Source: CAD feature listing. Evaluate the final solid. Frame: model axes, mm. A direction names the side the tool comes from. Coordinates: 2 decimals unless noted, no trailing zeros. Write each loop counter-clockwise with the first axis right and the second up, starting at its lowest first coordinate (ties: lowest second). Pieces come first, ordered by that corner, then holes. Notation, with made-up numbers: (-24.75, 11) -> (-20.75, 11) arc R17 cw to (-20.75, 40) -> close; hole circle Ø4 at (80.25, 82.5). An arc over 180 degrees is marked (long way). One line per item, written item: value. Start each with the question number.
1. Access query for faces 4 (the flat face through (25, 21, 0)), 5 (the flat face through (43, 31, 2)), 6 (the flat face through (46, 30, 35)). Directions: +Z, -Z, +X, -X, +Y, -Y. A direction counts if a zero-diameter tool reaches every point of the face in a straight line with its end or side. Return the directions, or none.
2. Section query C-C, the plane z = 10.65. Output: boundary loops of the cut face in (x, y) (3 decimals), and give its area (3 significant figures).
3. Section query D-D, the plane z = 3. Output: boundary loops of the cut face in (x, y).
4. Section query A-A, the plane y = 5.65. Output: boundary loops of the cut face in (x, z) (3 decimals).
5. Line query: line 1 (Z direction, x = 48.6, y = 5.65) (3 decimals); line 2 (Y direction, x = 48, z = 26); line 3 (Z direction, x = 7.5, y = 32). Output: solid intervals per line, ascending.
6. First-contact query: P1, Ø8, axis at y = 4.5, z = 40.5, coming from the -X side; P2, Ø12.5, axis at x = 18.5, y = 13.5, coming from the +Z side; P3, Ø3, axis at x = 42, y = 32.65, coming from the -Z side; P4, Ø1.7, axis at x = 4.5, y = 11, coming from the +Z side. Flat tips, straight axial feed; report the tip coordinate or a pass-through.
7. Mould query, pull axis Y, two halves, no side actions, for faces 1 (the cylindrical face through (47.97, 35.9, 40.21)), 2 (the cylindrical face through (48.03, 40.8, 45.87)), 3 (the flat face through (0, 21, 2)). Classes: released by +Y, released by -Y, zero draft, split by the parting line, or undercut.
8. Section query B-B, the plane x = 42. Output: boundary loops of the cut face in (y, z) (3 decimals), and give its area (4 significant figures).
from build123d import *

# Parameters (mm, degrees)
F0_W     = 50
F0_H     = 42.3
F0_R     = 2.8
F0_R_2   = 1.625
F1_DEPTH = 4
F2_R     = 2.8
F2_R_2   = 1.625
F3_DEPTH = 2
F4_W     = 4
F4_H     = 42.3
F5_DEPTH = 43.3
F6_R     = 12
F6_R_2   = 1.625
F7_DEPTH = 25
F8_R     = 5


with BuildPart() as f1:
    # F0 (on Top) → F1 (new body)
    with BuildSketch(Plane.XY):
        with Locations((25, 21.15)):
            Rectangle(F0_W, F0_H)
        with Locations((4, 9.65)):
            Circle(F0_R, mode=Mode.SUBTRACT)
        with Locations((42, 32.65)):
            Circle(F0_R, mode=Mode.SUBTRACT)
        with Locations((42, 32.65)):
            Circle(F0_R)
        with Locations((42, 32.65)):
            Circle(F0_R_2, mode=Mode.SUBTRACT)
        with Locations((4, 9.65)):
            Circle(F0_R)
        with Locations((4, 9.65)):
            Circle(F0_R_2, mode=Mode.SUBTRACT)
    extrude(amount=F1_DEPTH)

    # F2 (on face) → F3 (cut)
    with BuildSketch(Plane.XY.offset(4)):
        with Locations((4, 9.65)):
            Circle(F2_R)
        with Locations((4, 9.65)):
            Circle(F2_R_2, mode=Mode.SUBTRACT)
        with Locations((42, 32.65)):
            Circle(F2_R)
        with Locations((42, 32.65)):
            Circle(F2_R_2, mode=Mode.SUBTRACT)
    extrude(amount=-F3_DEPTH, mode=Mode.SUBTRACT)

    # F4 (on face) → F5 (join)
    with BuildSketch(Plane.XY.offset(4)):
        with Locations((48, 21.15)):
            Rectangle(F4_W, F4_H)
    extrude(amount=F5_DEPTH)

    # F6 (on face) → F7 (cut)
    with BuildSketch(Plane(origin=(46, 0, 0), x_dir=(0, -1, 0), z_dir=(-1, 0, 0))):
        with Locations((-21.15, 26.15)):
            Circle(F6_R)
        with Locations((-36.65, 41.65)):
            Circle(F6_R_2)
        with Locations((-5.65, 41.65)):
            Circle(F6_R_2)
        with Locations((-5.65, 10.65)):
            Circle(F6_R_2)
        with Locations((-36.65, 10.65)):
            Circle(F6_R_2)
    extrude(amount=-F7_DEPTH, mode=Mode.SUBTRACT)

    # F8
    f8_edges = [f1.edges().sort_by_distance(p)[0] for p in [
        (0, 0, 2),
        (0, 42.3, 2),
        (48, 42.3, 47.3),
        (48, 0, 47.3),
    ]]
    fillet(f8_edges, radius=F8_R)


solid = f1.part
Computed values:
1. face 4: -Z, +X, -X, +Y, -Y
1. face 5: +Z
1. face 6: +Z, -X, +Y, -Y
2. outline: (46, 0) -> (50, 0) -> (50, 4.025) -> (46, 4.025) -> close; (46, 7.275) -> (50, 7.275) -> (50, 35.025) -> (46, 35.025) -> close; (46, 38.275) -> (50, 38.275) -> (50, 42.3) -> (46, 42.3) -> close
2. area: 143 mm²
3. outline: (0, 5) arc R5 ccw to (5, 0) -> (50, 0) -> (50, 42.3) -> (5, 42.3) arc R5 ccw to (0, 37.3) -> close; hole circle Ø5.6 at (4, 9.65); hole circle Ø5.6 at (42, 32.65)
4. outline: (0, 0) -> (50, 0) -> (50, 9.025) -> (46, 9.025) -> (46, 4) -> (0, 4) -> close; (46, 12.275) -> (50, 12.275) -> (50, 40.025) -> (46, 40.025) -> close; (46, 43.275) -> (50, 43.275) -> (50, 47.3) -> (46, 47.3) -> close
5. line 1: z = 0 to 9.025, 12.275 to 40.025, 43.275 to 47.3
5. line 2: y = 0 to 9.15, 33.15 to 42.3
5. line 3: z = 0 to 4
6. P1: stops at x = 46
6. P2: stops at z = 4
6. P3: passes through
6. P4: stops at z = 2
7. face 1: undercut
7. face 2: released by +Y
7. face 3: zero draft
8. outline: (0, 0) -> (31.025, 0) -> (31.025, 2) -> (29.85, 2) -> (29.85, 4) -> (0, 4) -> close; (34.275, 0) -> (42.3, 0) -> (42.3, 4) -> (35.45, 4) -> (35.45, 2) -> (34.275, 2) -> close
8. area: 151.5 mm²
